Check sheet for the modelled part. Datum: model origin and axes. Units: mm. Give positions to 0.01 mm unless a question says otherwise; leave off trailing zeros. Order: outer loops, then holes, each group sorted by start corner. A loop starts at its lowest first (then second) coordinate and runs counter-clockwise, first axis right, second up. Notation, with made-up numbers: M 11,-3.75 L 19,-3.75 A25 ccw 19,21.25 Z; hole C -4,26 d11. An arc over 180 degrees is marked long. Answer in a Markdown table with one row per item. Add a question column.
from build123d import *

# Parameters (mm, degrees)
SKETCH_2_R         = 50
SKETCH_2_R_2       = 43
EXTRUDE_1_DEPTH    = 7.8
SKETCH_3_R         = 50
SKETCH_3_R_2       = 41.5
EXTRUDE_2_DEPTH    = 1
HOLE_WIZARD_M4_1_D = 3.3


with BuildPart() as part:
    # 草图2 → 凸台-拉伸1 (new body)
    with BuildSketch(Plane(origin=(0, 0, 0), x_dir=(1, 0, 0), z_dir=(0, 1, 0))):
        Circle(SKETCH_2_R)
        Circle(SKETCH_2_R_2, mode=Mode.SUBTRACT)
    extrude(amount=EXTRUDE_1_DEPTH)

    # 草图3 → 凸台-拉伸2 (add)
    with BuildSketch(Plane.XZ):
        Circle(SKETCH_3_R)
        Circle(SKETCH_3_R_2, mode=Mode.SUBTRACT)
    extrude(amount=EXTRUDE_2_DEPTH)

    # M4 螺纹孔1 (through all)
    with Locations(Plane(origin=(0, 7.8, 0), x_dir=(1, 0, 0), z_dir=(0, 1, 0))):
        with Locations((-32.880465325, 32.880465325), (-32.880465325, -32.880465325), (32.880465325, -32.880465325), (32.880465325, 32.880465325)):
            Hole(HOLE_WIZARD_M4_1_D / 2)


solid = part.part
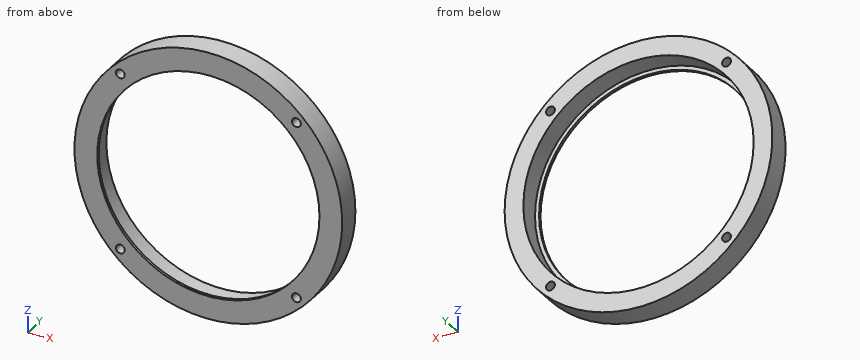
Q1. Go/stop test with flat-tipped pins: pin 1 (5 mm diameter, centred on y = 5.5, z = -9.5, fed in from +X); pin 2 (1.5 mm diameter, centred on y = 5, z = 9.5, fed in from +X); pin 3 (5 mm diameter, centred on y = 6.5, z = -6, fed in from -X). Record where each tip stops, or that it passes through.
Q2. Thickness scan on probe 1 along X at (y, z) = (5, 0); probe 2 along Z at (x, y) = (32, 7.75). Record the ranges inside material, lowest first.
Q3. Cross-section at C-C (y = 4.5). Record the boundary of the cut face in (x, z), and give its area (3 significant figures).
Q4. Cross-section at B-B (z = 0). Record the boundary of the cut face in (x, y), and give its area (3 significant figures).
Q5. Cross-section at A-A (x = 0). Record the boundary of the cut face in (y, z), and give its area (3 significant figures).
Values follow:
| question | item | result |
|---|---|---|
| 1 | pin 1 | x = 49.51 |
| 1 | pin 2 | x = 49.23 |
| 1 | pin 3 | x = -49.88 |
| 2 | probe 1 | -50 to -43, 43 to 50 |
| 2 | probe 2 | -38.42 to -34.28, -31.49 to -28.72, 28.72 to 31.49, 34.28 to 38.42 |
| 3 | outline | C 0,0 d100; hole C 0,0 d86; hole C -32.88,-32.88 d3.3; hole C -32.88,32.88 d3.3; hole C 32.88,-32.88 d3.3; hole C 32.88,32.88 d3.3 |
| 3 | area | 2,010 mm² |
| 4 | outline | M -50,-1 L -41.5,-1 L -41.5,0 L -43,0 L -43,7.8 L -50,7.8 Z; M 41.5,-1 L 50,-1 L 50,7.8 L 43,7.8 L 43,0 L 41.5,0 Z |
| 4 | area | 126 mm² |
| 5 | outline | M -1,-50 L 7.8,-50 L 7.8,-43 L 0,-43 L 0,-41.5 L -1,-41.5 Z; M -1,41.5 L 0,41.5 L 0,43 L 7.8,43 L 7.8,50 L -1,50 Z |
| 5 | area | 126 mm² |
